Autodesk Inventor part; units mm, degrees
ref_plane "Plan de construction1" through (-15, 0, -35) normal (1, 0, 0) x (0, 1, 0)
ref_plane "XZ Plane" through (0, 0, 0) normal (0, 1, 0) x (-1, 0, 0)
ref_plane "XY Plane" through (0, 0, 0) normal (0, 0, 1) x (1, 0, 0)
sketch "Esquisse1" plane through (0, 0, 0) normal (1, 0, 0) x (0, 1, 0)
  line L0 (9.5, 0) -> (9.5, -10)
  line L1 (0, 0) -> (0, -29.8331)
  line L2 (9.5, 0) -> (15, 0)
  line L3 (9.5, -10) -> (7.5, -10)
  line L4 (7.5, -10) -> (7.5, -15)
  line L5 (7.5, -15) -> (12, -25)
  line L6 (12, -25) -> (12, -70)
  line L7 (15, -70) -> (12, -70)
  line L8 (15, -70) -> (15, 0)
  dimension "d0" = 19
  dimension "d2" = 10
  dimension "d3" = 2
  dimension "d4" = 5
  dimension "d6" = 10
  dimension "d7" = 70
  dimension "d16" = 3
  dimension "d19" = 30
revolve "Révolution1" add sketch "Esquisse1" angle 360 about axis through (0, 0, 0) along (0, 0, -1)
chamfer "Chanfrein1" distance 5 distance2 7 1 edges at (0, -9.5, 0) measured on face at (-1.9544, 12.9294, 0)
chamfer "Chanfrein2" distance 2 angle 45 1 edges at (0, -12, -70)
ref_plane "Plan de construction1" through (-15, 0, -35) normal (1, 0, 0) x (0, 1, 0)
sketch "Esquisse3" plane through (-15, 0, -35) normal (1, 0, 0) x (0, 1, 0)
  circle A0 centre (0, 30) radius 3
  point P0 (0, 35)
  dimension "d23" = 6
  dimension "d24" = 5
extrude "Extrusion1" [suppressed]
sketch "Esquisse4" plane through (0, 0, 0) normal (1, 0, 0) x (0, 1, 0)
  line L0 (-15, 0) -> (15, 0)
  line L1 (-15, -70) -> (15, -70)
  line L2 (-9.5, -10) -> (-9.5, -7)
  line L3 (-9.5, -10) -> (9.5, -10)
  line L4 (-7.5, -15) -> (-7.5, -10)
  line L5 (-14.5, 0) -> (-9.5, -7)
  line L6 (-9.5, -7.9) -> (-11.8748, -8.7815)
  line L7 (-11.8748, -8.7815) -> (-9.5199, -12.0265)
  line L8 (-9.5199, -12.0265) -> (-8, -10)
  circle A0 centre (-9.5, -9.5) radius 1.5 construction
  line L9 (0, -72) -> (0, 12)
  point P0 (0, 0)
  dimension "d32" = 3
  dimension "d37" = 0.5
  dimension "d38" = 1.5
  dimension "d39" = 2.1
revolve "Révolution2" cut sketch "Esquisse4" angle 360 about axis through (0, 0, -10) along (0, 0, 1) contours L2 L3 L8 L7 L6
properties part number "cartridge_locker"
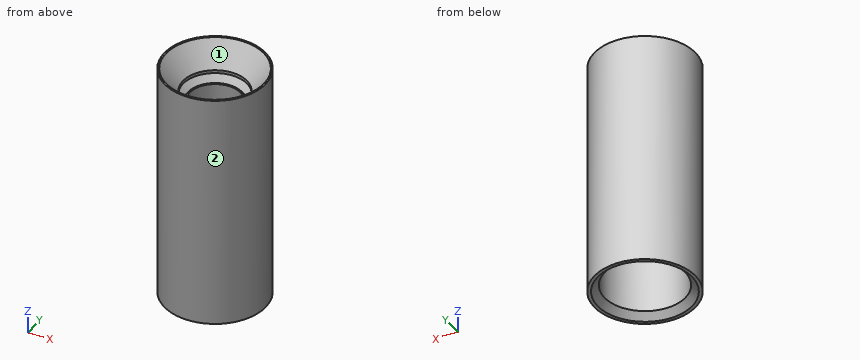
Input: part model. Units: mm. Frame: model coordinates. Face numbers are marked on the shaded views. Give positions to 0.01 mm unless a question says otherwise; leave off trailing zeros. Order: outer loops, then holes, each group sorted by start corner. A loop starts at its lowest first (then second) coordinate and runs counter-clockwise, first axis right, second up. Notation, with made-up numbers: (-36.75, -33.75) -> (-11.75, -33.75) arc R11 ccw to (-11.75, -16.75) -> close; hole circle Ø5 at (74.5, 30). An arc over 180 degrees is marked (long way). Use one line per item in the form item = value.
1) Section A-A, the plane x = 0. Return loops of the section in (y, z).
Response values:
outline = (-15, -70) -> (-14, -70) -> (-12, -68) -> (-12, -25) -> (-7.5, -15) -> (-7.5, -10) -> (-8, -10) -> (-9.52, -12.03) -> (-11.87, -8.78) -> (-9.5, -7.9) -> (-9.5, -7) -> (-14.5, 0) -> (-15, 0) -> close; (7.5, -15) -> (12, -25) -> (12, -68) -> (14, -70) -> (15, -70) -> (15, 0) -> (14.5, 0) -> (9.5, -7) -> (9.5, -7.9) -> (11.87, -8.78) -> (9.52, -12.03) -> (8, -10) -> (7.5, -10) -> close
2) Mould query, pull axis X, two halves, no side actions, for the marked faces 1 and 2. Classes: pulls with the +X half, pulls with the -X half, needs draft (parallel to the pull), parting line crosses it, or undercut.
Response values:
face_1 = undercut
face_2 = parting line crosses it
3) Line query: probe 1 along Y at (x, z) = (0.5, -38.5); probe 2 along X at (y, z) = (0, -12.2); probe 3 along X at (y, z) = (0, -45.5). Output: solid intervals per line, ascending.
Response values:
probe_1 = -14.99 to -11.99, 11.99 to 14.99
probe_2 = -15 to -7.5, 7.5 to 15
probe_3 = -15 to -12, 12 to 15
4) First-contact query: pin 1 Ø10 at (x, y) = (3, 11) entering from +Z; pin 2 Ø1 at (y, z) = (-2.5, -55) entering from -X; pin 3 Ø1 at (x, z) = (1, -59) entering from -Y; pin 4 Ø8 at (y, z) = (12, -45) entering from +X. Flat tips, straight axial feed; report the tip coordinate or a pass-through.
Response values:
pin_1 = 0
pin_2 = -14.87
pin_3 = -14.99
pin_4 = 12.69
5) Section C-C, the plane z = -26. Return loops of the section in (x, y).
Response values:
outline = circle Ø30 at (0, 0); hole circle Ø24 at (0, 0)
